from build123d import *

# Parameters (mm, degrees)
F0_R     = 1.5875
F0_R_2   = 3.254514
F0_R_3   = 3.175
F1_DEPTH = 25.4


with BuildPart() as f1:
    # F0 (on Front) → F1 (new body)
    with BuildSketch(Plane.XZ):
        with BuildLine():
            ThreePointArc((9.524938, 56.923091), (-0.27613, 47.436536), (-9.510924, 57.475173))
            Line((-9.510924, 57.475173), (-15.775539, 1.774256))
            ThreePointArc((-15.775539, 1.774256), (-0.006833, 15.874999), (15.774006, 1.787837))
            Line((15.774006, 1.787837), (9.524938, 56.923091))
        make_face()
        with Locations((-1.5875, 39.808989)):
            Circle(F0_R, mode=Mode.SUBTRACT)
        with BuildLine():
            ThreePointArc((15.774006, 1.787837), (-0.006833, 15.874999), (-15.775539, 1.774256))
            ThreePointArc((-15.775539, 1.774256), (-15.875, 0), (-15.775539, -1.774256))
            ThreePointArc((-15.775539, -1.774256), (-0.006834, -15.874999), (15.774006, -1.787837))
            ThreePointArc((15.774006, -1.787837), (15.849731, -0.895344), (15.875, 0))
            ThreePointArc((15.875, 0), (15.849731, 0.895343), (15.774006, 1.787837))
        make_face()
        Circle(F0_R_2, mode=Mode.SUBTRACT)
        with BuildLine():
            ThreePointArc((15.774006, -1.787837), (-0.006834, -15.874999), (-15.775539, -1.774256))
            Line((-15.775539, -1.774256), (-9.574969, -56.905723))
            ThreePointArc((-9.574969, -56.905723), (-6.621351, -50.412213), (0, -47.757548))
            ThreePointArc((0, -47.757548), (0.353832, -47.764081), (0.707181, -47.783671))
            ThreePointArc((0.707181, -47.783671), (6.775215, -50.562558), (9.558309, -56.628662))
            ThreePointArc((9.558309, -56.628662), (9.578269, -56.98532), (9.584925, -57.342473))
            ThreePointArc((9.584925, -57.342473), (6.902424, -63.992835), (0.356407, -66.920769))
            Line((0.356407, -66.920769), (44.452102, -65.279972))
            ThreePointArc((44.452102, -65.279972), (36.513833, -57.196991), (44.743016, -49.410383))
            Line((44.743016, -49.410383), (22.371508, -48.583965))
            ThreePointArc((22.371508, -48.583965), (13.670923, -42.795517), (12.300367, -32.435599))
            Line((12.300367, -32.435599), (15.774006, -1.787837))
        make_face()
        with BuildLine():
            ThreePointArc((44.743016, -49.410383), (36.513833, -57.196991), (44.452102, -65.279972))
            ThreePointArc((44.452102, -65.279972), (50.063403, -62.954389), (52.3875, -57.342473))
            ThreePointArc((52.3875, -57.342473), (50.165318, -51.834384), (44.743016, -49.410383))
        make_face()
        with Locations((44.45, -57.342473)):
            Circle(F0_R_3, mode=Mode.SUBTRACT)
        with BuildLine():
            ThreePointArc((0, -47.757548), (-6.621351, -50.412213), (-9.574969, -56.905723))
            ThreePointArc((-9.574969, -56.905723), (-6.805935, -64.091549), (0.356407, -66.920769))
            ThreePointArc((0.356407, -66.920769), (6.902424, -63.992835), (9.584925, -57.342473))
            Line((9.584925, -57.342473), (9.477405, -57.342473))
            Line((9.477405, -57.342473), (9.558309, -56.628662))
            ThreePointArc((9.558309, -56.628662), (6.775215, -50.562558), (0.707181, -47.783671))
            Line((0.707181, -47.783671), (0, -47.757548))
        make_face()
        with Locations((0, -57.342473)):
            Circle(F0_R_3, mode=Mode.SUBTRACT)
        with BuildLine():
            ThreePointArc((9.524938, 56.923091), (9.524984, 56.940312), (9.525, 56.957532))
            ThreePointArc((9.525, 56.957532), (0.258916, 66.479013), (-9.510924, 57.475173))
            ThreePointArc((-9.510924, 57.475173), (-0.27613, 47.436536), (9.524938, 56.923091))
        make_face()
        with Locations((0, 56.957532)):
            Circle(F0_R_3, mode=Mode.SUBTRACT)
    extrude(amount=F1_DEPTH)


solid = f1.part
Read the model definition and answer for the solid it produces. Units are mm, in the model's axes. A direction names the side the tool comes from. Coordinates: 2 decimals unless noted, no trailing zeros. Loops run counter-clockwise (first coordinate to the right, second up) from the corner with the lowest first, then second, coordinate; pieces in that order, holes last.
Q1. Each of these flat-tipped pins is pushed along its axis until it touches: pin 1 Ø10 at (y, z) = (-3.5, -17.5) entering from -X; pin 2 Ø3 at (x, z) = (-1.59, 39.81) entering from +Y; pin 3 Ø8 at (y, z) = (-8, -42) entering from +X; pin 4 Ø1 at (x, y) = (28.5, -20) entering from -Z. Where does it stop, or does it pass through?
Q2. The part is cut by section B-B on y = -13.5. Give the number of separate pieces and of enclosed holes in the cut face, and give its area (3 significant figures).
Q3. Which of the six approach directions +Z, -Z, +X, -X, +Y, -Y give full straight-line access (tool end or side, diameter ignored) to faces 1 (the face through (0.46, -12.52, 66.47)), 2 (the face through (14.013, -12.522, -17.326))?
Q4. The part is cut by section C-C on z = -5.5. Write down the section's boundary in (x, y), and give its area (3 significant figures).
Q5. The part is cut by section D-D on x = -7. Write down the section's boundary in (y, z), and give its area (3 significant figures).
Q6. Consider probe 1 along Z at (x, y) = (44.45, -8.75); probe 2 along Z at (x, y) = (43.5, -21); probe 3 along X at (y, z) = (-4.5, 56.5). Determine where each line is inside the solid, lowest interval first.
Q7. The mould has two halves that part along Z. Classify faces 3 (the face through (-15.875, -12.522, 0.025)), 4 (the face through (3, 0, -14)), 5 (the face through (22.1, -12.52, -66.11)), 6 (the face through (3.104, -12.522, 0.978)): +Z half, -Z half, draft (parallel to the pull), parting line (faces both ways), or undercut.
Q8. The part is cut by section A-A on x = 43. Write down the section's boundary in (y, z).
Results below:
1. pin 1: stops at x = -14.57
1. pin 2: passes through
1. pin 3: stops at x = 16.53
1. pin 4: stops at z = -65.89
2. separate pieces: 1
2. enclosed holes: 7
2. area: 3,810 mm2
3. face 1: +Z, +Y, -Y
3. face 2: +X, +Y, -Y
4. outline: (-15.36, -25.4) - (15.35, -25.4) - (15.35, 0) - (-15.36, 0) - close
4. area: 780 mm2
5. outline: (-25.4, -63.89) - (0, -63.89) - (0, 63.42) - (-25.4, 63.42) - close
5. area: 3,230 mm2
6. probe 1: z = -65.28 to -60.52, -54.17 to -49.4
6. probe 2: z = -65.32 to -60.37, -54.31 to -49.36
6. probe 3: x = -9.62 to -3.14, 3.14 to 9.57
7. face 3: parting line
7. face 4: draft
7. face 5: -Z half
7. face 6: undercut
8. outline: (-25.4, -65.33) - (0, -65.33) - (0, -60.17) - (-25.4, -60.17) - close; (-25.4, -54.52) - (0, -54.52) - (0, -49.35) - (-25.4, -49.35) - close
